Input: part model. Units: mm. Frame: model coordinates. A direction names the side the tool comes from. Give positions to 0.01 mm unless a question says otherwise; leave off trailing zeros. Order: outer loops, then holes, each group sorted by start corner. A loop starts at its lowest first (then second) coordinate and runs counter-clockwise, first axis right, second up. Notation, with made-up numbers: (49.5, 0.5) -> (53.5, 0.5) arc R32 cw to (53.5, 34.5) -> close; hole circle Ø3 at (-10.75, 32). An arc over 180 degrees is marked (long way). Use a Markdown table: item, result. Add a question column.
Autodesk Inventor part; units mm, degrees
ref_plane "YZ Plane" through (0, 0, 0) normal (1, 0, 0) x (0, 1, 0)
ref_plane "XZ Plane" through (0, 0, 0) normal (0, 1, 0) x (-1, 0, 0)
ref_plane "XY Plane" through (0, 0, 0) normal (0, 0, 1) x (1, 0, 0)
sketch "Skizze1" plane through (0, 0, 0) normal (0, 0, 1) x (1, 0, 0)
  line L0 (-9.02, 0) -> (54.12, 0)
  line L1 (0, -4.06) -> (0, 24.36)
  line L2 (0, 0) -> (45.1, 0)
  line L3 (45.1, 0) -> (45.1, 20.3)
  line L4 (45.1, 20.3) -> (0, 20.3)
  line L5 (0, 20.3) -> (0, 0)
  point P0 (0, 20.3)
  dimension "d0" = 20.3
  dimension "d1" = 45.1
extrude "Extrusion1" add sketch "Skizze1" along normal blind 3.5
sketch "Skizze2" plane through (0, 0, 3.5) normal (0, 0, 1) x (1, 0, 0)
  circle A0 centre (35.4, 10.2) radius 7.9
  circle A1 centre (9.7, 10.2) radius 7.9
  line L0 (0, 20.3) -> (0, 0)
  line L1 (0, 0) -> (45.1, 0)
  dimension "d4" = 15.8
  dimension "d5" = 15.8
  dimension "d6" = 25.7
  dimension "d8" = 9.7
  dimension "d9" = 10.2
  dimension "d10" = 10.2
extrude "Extrusion2" add sketch "Skizze2" along normal blind 12.1
sketch "Skizze3" plane through (0, 0, 0) normal (0, 0, -1) x (-1, 0, 0)
  line L0 (-17.55, 2.7) -> (-27.55, 2.7)
  line L1 (-27.55, 2.7) -> (-27.55, 0.4)
  line L2 (-27.55, 0.4) -> (-17.55, 0.4)
  line L3 (-17.55, 0.4) -> (-17.55, 2.7)
  line L4 (0, 0) -> (-45.1, 0)
  line L5 (-45.1, 0) -> (-45.1, 20.3)
  dimension "d13" = 2.7
  dimension "d14" = 2.3
  dimension "d17" = 10
  dimension "d18" = 17.55
extrude "Extrusion3" add sketch "Skizze3" along normal blind 4
properties part number "Sensor_Dummy"
Q1. Section query A-A (x = 26.5). Return loops of the section in (y, z), plus the area to 4 significant figures.
Q2. First-contact query: pin 1 (3 mm diameter, centred on x = 29.5, z = 5.5, fed in from +Y); pin 2 (0.7 mm diameter, centred on y = 2, z = -2.5, fed in from -X); pin 3 (4 mm diameter, centred on x = 11, y = 4.5, fed in from -Z). Flat tips, straight axial feed; report the tip coordinate or a pass-through.
Q3. Section query C-C (z = 5.5). Return loops of the section in (x, y), plus the area to 3 significant figures.
Q4. Section query B-B (y = 10.2). Return loops of the section in (x, z), plus the area to 3 significant figures.
Q5. Section query D-D (z = -1.5). Return loops of the section in (x, y).
Q6. Ray query, line 1 (Z direction, x = 42, y = 14.75); line 2 (X direction, y = 16.25, z = 5.25); line 3 (Y direction, x = 24, z = -1.5). Return the intervals inside material, ascending.
Q7. Access query for faces 1 (the cylindrical face through (16.998, 13.226, 9.465)), 2 (the flat face through (23, 0.4, -2)), 3 (the flat face through (22, 2.7, -2)). Directions: +Z, -Z, +X, -X, +Y, -Y. A direction counts if a zero-diameter tool reaches every point of the face in a straight line with its end or side. Return the directions, or none.
Solution:
| question | item | result |
|---|---|---|
| 1 | outline | (0, 0) -> (0.4, 0) -> (0.4, -4) -> (2.7, -4) -> (2.7, 0) -> (20.3, 0) -> (20.3, 3.5) -> (0, 3.5) -> close |
| 1 | area | 80.25 mm² |
| 2 | pin 1 | stops at y = 16.76 |
| 2 | pin 2 | stops at x = 17.55 |
| 2 | pin 3 | stops at z = 0 |
| 3 | outline | circle Ø15.8 at (9.7, 10.2); circle Ø15.8 at (35.4, 10.2) |
| 3 | area | 392 mm² |
| 4 | outline | (0, 0) -> (45.1, 0) -> (45.1, 3.5) -> (43.3, 3.5) -> (43.3, 15.6) -> (27.5, 15.6) -> (27.5, 3.5) -> (17.6, 3.5) -> (17.6, 15.6) -> (1.8, 15.6) -> (1.8, 3.5) -> (0, 3.5) -> close |
| 4 | area | 540 mm² |
| 5 | outline | (17.55, 0.4) -> (27.55, 0.4) -> (27.55, 2.7) -> (17.55, 2.7) -> close |
| 6 | line 1 | z = 0 to 3.5 |
| 6 | line 2 | x = 4.62 to 14.78, 30.32 to 40.48 |
| 6 | line 3 | y = 0.4 to 2.7 |
| 7 | face 1 | +Z |
| 7 | face 2 | -Z, +X, -X, -Y |
| 7 | face 3 | -Z, +X, -X, +Y |
